Can you work these out from the model? Positions are in its coordinate system, mm. A direction names the side the tool comes from. Give positions to 0.01 mm unless a question says otherwise; leave off trailing zeros. Order: outer loops, then holes, each group sorted by start corner. A loop starts at its lowest first (then second) coordinate and runs counter-clockwise, first axis right, second up. Notation, with made-up numbers: M -26.5,-10.75 L -12.5,-10.75 A22 ccw -12.5,7.25 Z; hole C 28.25,7 d4. An arc over 180 degrees is marked long. Use a Markdown table: item, result. Add a question column.
Autodesk Inventor part; units mm, degrees
ref_plane "YZ Plane" through (0, 0, 0) normal (1, 0, 0) x (0, 1, 0)
ref_plane "XZ Plane" through (0, 0, 0) normal (0, 1, 0) x (-1, 0, 0)
ref_plane "XY Plane" through (0, 0, 0) normal (0, 0, 1) x (1, 0, 0)
sketch "Sketch1" plane through (0, 0, 0) normal (0, 1, 0) x (-1, 0, 0)
  line L0 (0, 0) -> (40, 0)
  line L1 (40, 0) -> (40, -20)
  line L2 (40, -20) -> (0, -20)
  line L3 (0, -20) -> (0, 0)
  dimension "d0" = 40
  dimension "d1" = 20
extrude "Extrusion1" add sketch "Sketch1" along normal blind 6
sketch "Sketch2" plane through (0, 6, 0) normal (0, 1, 0) x (1, 0, 0)
  line L0 (0, 0) -> (6, 0)
  line L1 (6, 0) -> (6, 20)
  line L2 (6, 20) -> (0, 20)
  line L3 (0, 20) -> (0, 0)
  dimension "d4" = 6
  dimension "d5" = 20
extrude "Extrusion2" add sketch "Sketch2" against normal blind 30
fillet "Fillet1" radius 5 1 edges at (0, 0, -10)
fillet "Fillet4" radius 5 1 edges at (6, 6, -10)
sketch "Sketch5" plane through (0, 0, 0) normal (0, -1, 0) x (1, 0, 0)
  circle A0 centre (-24, -10) radius 3
  line L0 (-40, -20) -> (-40, 0)
  line L1 (-5, -20) -> (-40, -20)
  line L2 (6, -20) -> (6, 0)
  circle A1 centre (-44, -10) radius 3
  line L3 (-40, 0) -> (-5, 0)
  point P0 (0, 0)
  dimension "d18" = 6
  dimension "d20" = 10
  dimension "d47" = 30
  dimension "d48" = 6
  dimension "d49" = 20
  dimension "d50" = 10
fillet "Fillet7" radius 2 2 edges at (-40, 3, 0) (-40, 3, -20)
sketch "Sketch8" plane through (0, -24, -20) normal (-1, 0, 0) x (0, 0, 1)
  line L0 (20, 0) -> (0, 0)
  line L1 (0, 0) -> (20, 0)
  line L2 (20, 0) -> (20, -6)
  line L3 (20, -6) -> (0, -6)
  line L4 (0, -6) -> (0, 0)
  point P0 (20, 24)
  dimension "d35" = 6
extrude "Extrusion6" add sketch "Sketch8" against normal blind 30
fillet "Fillet8" radius 5 1 edges at (0, -30, -10)
fillet "Fillet9" radius 5 1 edges at (6, -24, -10)
sketch "Sketch9" plane through (30, -24, 0) normal (0, 1, 0) x (1, 0, 0)
  line L0 (0, 20) -> (0, 0)
  line L1 (0, 20) -> (-6, 20)
  line L2 (-6, 20) -> (-6, 0)
  line L3 (-6, 0) -> (0, 0)
  line L4 (0, 0) -> (0, 20)
  point P0 (-30, 0)
  dimension "d40" = 6
  dimension "d41" = 20
extrude "Extrusion7" add sketch "Sketch9" along normal blind 10
fillet "Fillet10" radius 5 1 edges at (24, -24, -10)
fillet "Fillet11" radius 5 1 edges at (30, -30, -10)
fillet "Fillet12" radius 3 2 edges at (24, -14, -10) (30, -14, -10)
extrude "Extrusion8" cut sketch "Sketch5" against normal through all both and the other way through all
properties part number "Cable_Guide_Holder"
1. I need wall thicknesses on L1, parallel to Z at x = -24, y = 2; L2, parallel to X at y = -22, z = -3.5; L3, parallel to Y at x = 11, z = -5. Which ranges of each line are inside material? Lowest first, please. Write a range as [from, to].
2. If we section it at B-B, the plane y = -16: List the corners of the cut face in (x, z) for me.
3. Will these pins go through, and if not, where does the flat tip stop? pin 1 (1 mm diameter, centred on y = -20, z = -12, fed in from -X); pin 2 (1 mm diameter, centred on y = -3.5, z = -3.5, fed in from -X); pin 3 (10 mm diameter, centred on x = -20.5, z = -9.5, fed in from -Y).
4. On a 3-axis mill with a long thin cutter (end or side, diameter ignored), from which of +Z, -Z, +X, -X, +Y, -Y can I reach the whole of each face in a straight line? I mean faces 1 (the face through (4, 5, -10)), 2 (the face through (6, -9, -10)), 3 (the face through (0, -15, -10)). Say none if no direction works.
5. If we section it at C-C, the plane x = -24: List the corners of the cut face in (y, z) for me, then the cut area to 3 significant figures.
6. We'd pull the mould along Z, two halves only. Please class faces 4 (the face through (-27, 3, -10)), 5 (the face through (-39.43, 3.04, -0.6)), 6 (the face through (30, -21, -10)): +Z half, -Z half, draft (parallel to the pull), parting line (faces both ways), or undercut.
Geometry results:
| question | item | result |
|---|---|---|
| 1 | L1 | z = [-20, -13], [-7, 0] |
| 1 | L2 | x = [0, 7], [23, 30] |
| 1 | L3 | y = [-30, -24] |
| 2 | outline | M 0,-20 L 6,-20 L 6,0 L 0,0 Z; M 24.17,-20 L 29.83,-20 L 29.83,0 L 24.17,0 Z |
| 3 | pin 1 | stops at x = 0 |
| 3 | pin 2 | stops at x = -0.42 |
| 3 | pin 3 | stops at y = 0 |
| 4 | face 1 | +Z, -Z, +X, +Y |
| 4 | face 2 | +Z, -Z, +Y |
| 4 | face 3 | +Z, -Z, -X, -Y |
| 5 | outline | M 0,-20 L 6,-20 L 6,-13 L 0,-13 Z; M 0,-7 L 6,-7 L 6,0 L 0,0 Z |
| 5 | area | 84.0 mm^2 |
| 6 | face 4 | undercut |
| 6 | face 5 | +Z half |
| 6 | face 6 | draft |
